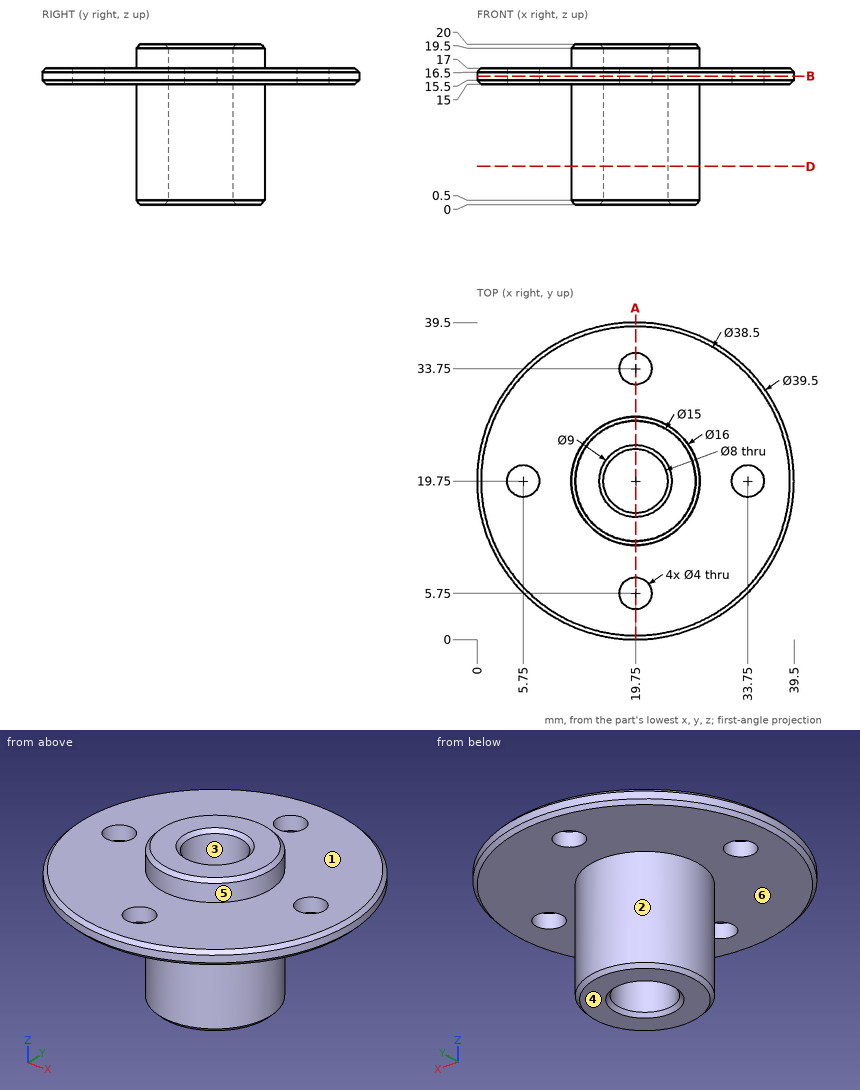
Study the drawing (mm; zero at the part's minimum x, y, z) and answer. A direction names the side the tool comes from. Round coordinates to 2 decimals unless told otherwise and drop trailing zeros. Write each loop counter-clockwise with the first axis right and the second up, starting at its lowest first coordinate (ties: lowest second). Pieces come first, ordered by that corner, then holes.
1) A cutting plane is placed at A-A on x = 19.75. Give the number of separate pieces and of enclosed holes in the cut face, and give its area (4 significant figures).
2) A cutting plane is placed at B-B on z = 16. Determine the outline of the cut face in (x, y).
3) A cutting plane is placed at D-D on z = 4.75. Determine the outline of the cut face in (x, y).
4) Which of the six approach directions +Z, -Z, +X, -X, +Y, -Y give full straight-line access (tool end or side, diameter ignored) to the marked faces 4, 5 and 6?
5) Determine the mould class of the marked faces 1, 2 and 3 for opening direction Y: pulls with the +Y half, pulls with the -Y half, needs draft (parallel to the pull), parting line crosses it, or undercut.
6) Flat-ended cylindrical pins translate along their axes: P1, Ø3.5, axis at x = 19.75, y = 5.75, coming from the +Z side; P2, Ø6, axis at x = 31.5, y = 26.5, coming from the -Z side; P3, Ø6, axis at y = 35, z = 12.5, coming from the +X side; P4, Ø1.5, axis at x = 15.5, z = 3.5, coming from the -Y side. Find the tip coordinate at first contact, or state that the pin passes through.
7) Consider probe 1 along Y at (x, z) = (19.75, 15.85); probe 2 along Z at (x, y) = (11, 15); probe 3 along Y at (x, z) = (33.75, 16.4). Determine where each line is inside the solid, lowest interval first.
Entries:
1. separate pieces: 4
1. enclosed holes: 0
1. area: 189.5 mm2
2. outline: circle Ø39.5 at (19.75, 19.75); hole circle Ø4 at (5.75, 19.75); hole circle Ø8 at (19.75, 19.75); hole circle Ø4 at (19.75, 5.75); hole circle Ø4 at (19.75, 33.75); hole circle Ø4 at (33.75, 19.75)
3. outline: circle Ø16 at (19.75, 19.75); hole circle Ø8 at (19.75, 19.75)
4. face 4: -Z, +X, -X, +Y, -Y
4. face 5: +Z
4. face 6: -Z
5. face 1: needs draft
5. face 2: parting line crosses it
5. face 3: undercut
6. P1: passes through
6. P2: stops at z = 15
6. P3: stops at x = 33.38
6. P4: stops at y = 12.56
7. probe 1: y = 0 to 3.75, 7.75 to 15.75, 23.75 to 31.75, 35.75 to 39.5
7. probe 2: z = 15 to 17
7. probe 3: y = 5.82 to 17.75, 21.75 to 33.68
